Design review of the part built by this model. Coordinates are the model's own, in mm. A direction names the side the tool comes from. Coordinates: 2 decimals unless noted, no trailing zeros. Loops run counter-clockwise (first coordinate to the right, second up) from the corner with the lowest first, then second, coordinate; pieces in that order, holes last. Notation, with made-up numbers: (74, -19.75) - (107, -19.75) arc R6 ccw to (107, -12.75) - close; hole circle Ø3 at (-16, -37.75). An arc over 180 degrees is marked (long way). Answer in a Markdown table with one row per item. Add a question column.
(1) We need section A-A, the plane y = 10.5. Write out the cut boundary in (x, z).
(2) To check wall thickness, follow L1, parallel to X at y = 13, z = -5.5; L2, parallel to Z at x = 31.5, y = 18.25; L3, parallel to Y at x = 30, z = 2. State the ranges of each line that lie inside material, in increasing order. Write a range as [from, to].
(3) The part is to be moulded in two halves that separate along X. For faces 3 (the face through (38, 14, 0)), 4 (the face through (40, 11, -1)), 5 (the face through (20, 11, -36.5)), say which applies: released by +X, released by -X, zero draft, split by the parting line, or undercut.
(4) Clearance check with flat-ended pins moving along their axes: pin 1 (2 mm diameter, centred on x = 31, z = 15, fed in from +Y); pin 2 (7 mm diameter, centred on y = 12.5, z = 7.5, fed in from -X); pin 3 (12 mm diameter, centred on x = 27, z = -28, fed in from +Y); pin 4 (2 mm diameter, centred on x = 35.5, y = 8.5, fed in from -Z). State where each tip first meets the part, or that it passes through.
(5) We need section D-D, the plane x = 20. Write out the cut boundary in (y, z).
(6) We need section C-C, the plane z = -20.5. Write out the cut boundary in (x, y).
(7) We need section B-B, the plane x = 10. Write out the cut boundary in (y, z).
(8) For faces 1 (the face through (3, 7, 0)), 2 (the face through (1, 21, 0)), list the 3-axis set-ups (+Z, -Z, +X, -X, +Y, -Y) from which the entire face can be reached by the end or side of a thin tool; tool diameter is ignored.
Autodesk Inventor part; units mm, degrees
ref_plane "YZ Plane" through (0, 0, 0) normal (1, 0, 0) x (0, 1, 0)
ref_plane "XZ Plane" through (0, 0, 0) normal (0, 1, 0) x (-1, 0, 0)
ref_plane "XY Plane" through (0, 0, 0) normal (0, 0, 1) x (1, 0, 0)
sketch "Esquisse1" plane through (0, 0, 0) normal (0, 0, 1) x (1, 0, 0)
  line L0 (0, 21) -> (40, 21)
  line L1 (40, 21) -> (40, 0)
  line L2 (40, 0) -> (0, 0)
  line L3 (0, 0) -> (0, 21)
  line L4 (-8, 0) -> (48, 0)
  line L5 (0, -4.2) -> (0, 25.2)
  point P0 (0, 0)
  dimension "d0" = 40
  dimension "d1" = 21
extrude "Extrusion1" add sketch "Esquisse1" along normal mid plane 73
sketch "Esquisse2" plane through (0, 0, 36.5) normal (0, 0, 1) x (1, 0, 0)
  circle A0 centre (10, 10.5) radius 7
  circle A1 centre (30, 10.5) radius 7
  line L0 (40, 21) -> (0, 21)
  line L1 (0, 21) -> (0, 0)
  line L2 (40, 0) -> (40, 21)
  line L3 (0, 0) -> (40, 0)
  dimension "d4" = 14
  dimension "d5" = 14
  dimension "d11" = 10.5
  dimension "d20" = 10.5
  dimension "d21" = 20
extrude "Extrusion2" cut sketch "Esquisse2" against normal through all contours A0 | A1
sketch "Esquisse3" plane through (0, 21, 36.5) normal (0, 1, 0) x (1, 0, 0)
  line L0 (2, 71) -> (38, 71)
  line L1 (38, 71) -> (38, 2)
  line L2 (38, 2) -> (2, 2)
  line L3 (2, 2) -> (2, 71)
  line L4 (0, 73) -> (40, 73)
  line L5 (40, 0) -> (0, 0)
  line L6 (40, 73) -> (40, 0)
  line L7 (0, 73) -> (0, 0)
  point P0 (0, 36.5)
  dimension "d14" = 2
  dimension "d15" = 2
  dimension "d16" = 2
  dimension "d17" = 2
extrude "Extrusion3" cut sketch "Esquisse3" against normal blind 14 contours L0 L1 L2 L3
equation "\"d5\" = d4"
equation "\"d11\" = d20"
equation "\"d15\" = d14"
equation "\"d16\" = d15"
equation "\"d17\" = d16"
properties part number "support pile"
Responses:
| question | item | result |
|---|---|---|
| 1 | outline | (0, -36.5) - (3, -36.5) - (3, -34.5) - (2, -34.5) - (2, 34.5) - (3, 34.5) - (3, 36.5) - (0, 36.5) - close; (17, -36.5) - (23, -36.5) - (23, -34.5) - (17, -34.5) - close; (17, 34.5) - (23, 34.5) - (23, 36.5) - (17, 36.5) - close; (37, -36.5) - (40, -36.5) - (40, 36.5) - (37, 36.5) - (37, 34.5) - (38, 34.5) - (38, -34.5) - (37, -34.5) - close |
| 2 | L1 | x = [0, 2], [38, 40] |
| 2 | L2 | z = [-36.5, -34.5], [34.5, 36.5] |
| 2 | L3 | y = [0, 3.5] |
| 3 | face 3 | undercut |
| 3 | face 4 | released by +X |
| 3 | face 5 | zero draft |
| 4 | pin 1 | stops at y = 3.79 |
| 4 | pin 2 | stops at x = 0 |
| 4 | pin 3 | stops at y = 7 |
| 4 | pin 4 | passes through |
| 5 | outline | (0, -36.5) - (21, -36.5) - (21, -34.5) - (7, -34.5) - (7, 34.5) - (21, 34.5) - (21, 36.5) - (0, 36.5) - close |
| 6 | outline | (0, 0) - (40, 0) - (40, 21) - (38, 21) - (38, 7) - (36.06, 7) arc R7 cw to (23.94, 7) - (16.06, 7) arc R7 cw to (3.94, 7) - (2, 7) - (2, 21) - (0, 21) - close |
| 7 | outline | (0, -36.5) - (3.5, -36.5) - (3.5, 36.5) - (0, 36.5) - close; (17.5, -36.5) - (21, -36.5) - (21, -34.5) - (17.5, -34.5) - close; (17.5, 34.5) - (21, 34.5) - (21, 36.5) - (17.5, 36.5) - close |
| 8 | face 1 | +Y |
| 8 | face 2 | +Z, -Z, +X, -X, +Y |
